Check sheet for the drawn part. Datum: minimum x, y, z corner. Units: mm. A direction names the side the tool comes from. Round coordinates to 2 decimals unless told otherwise and drop trailing zeros. Write each loop counter-clockwise with the first axis right and the second up, starting at its lowest first coordinate (ties: lowest second). Pieces come first, ordered by that corner, then holes.
Item 1: Cross-section at A-A on x = 12.75. Enter the section's corners in (y, z).
Item 2: Cross-section at B-B on z = 0.2. Enter the section's corners in (x, y).
Item 3: Tool access check on the marked faces 1 and 2. Record the directions out of +Z, -Z, +X, -X, +Y, -Y that give a thin tool (end or side, any length) a straight path to the whole face; none if there is none.
Item 4: Cross-section at C-C on y = 3.5. Enter the section's corners in (x, z).
Item 5: Release check for a two-part mould opening along Y. For the marked faces 3, 4 and 5 record: +Y half, -Y half, draft (parallel to the pull), parting line (faces both ways), or undercut.
Item 6: Cross-section at D-D on x = 9. Enter the section's corners in (y, z).
Item 7: Material ranges on line 1 (X direction, y = 11, z = 1.05); line 2 (Y direction, x = 12.5, z = 0.3); line 3 (Y direction, x = 8.25, z = 0.25), recorded low to high.
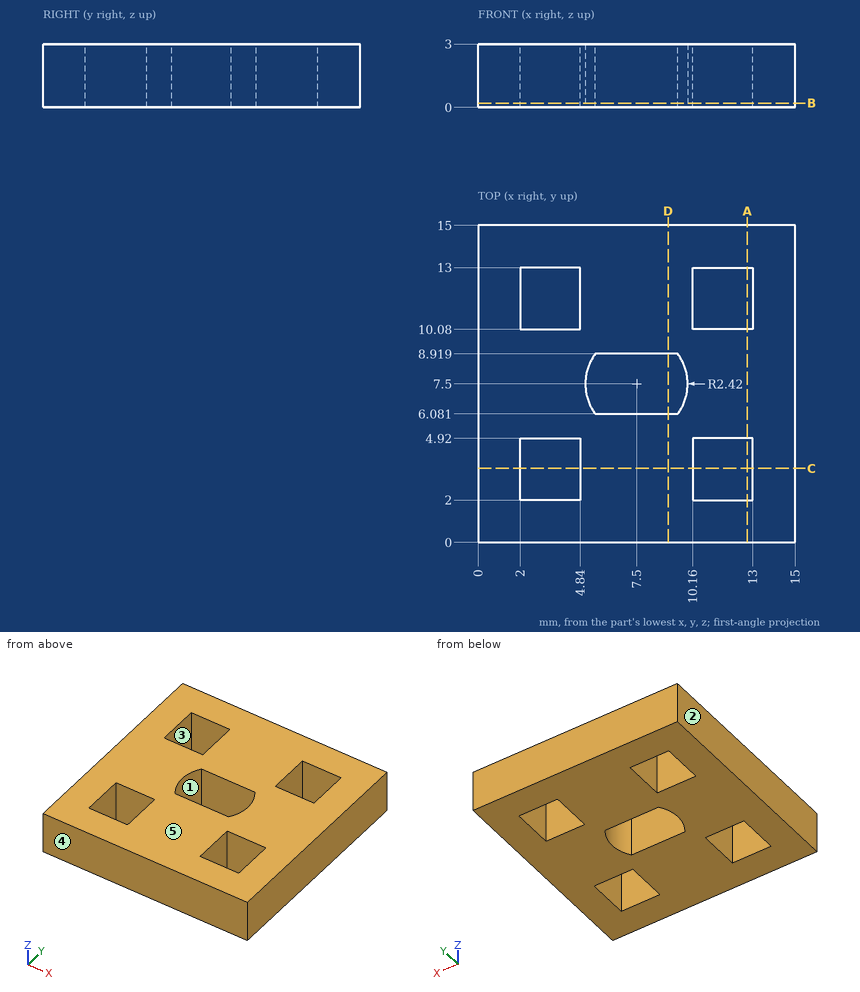
Response values:
1. outline: (0, 0) - (2, 0) - (2, 3) - (0, 3) - close; (4.92, 0) - (10.08, 0) - (10.08, 3) - (4.92, 3) - close; (13, 0) - (15, 0) - (15, 3) - (13, 3) - close
2. outline: (0, 0) - (15, 0) - (15, 15) - (0, 15) - close; hole (2, 2) - (4.84, 2) - (4.84, 4.92) - (2, 4.92) - close; hole (2, 10.08) - (4.84, 10.08) - (4.84, 13) - (2, 13) - close; hole (5.54, 6.08) - (9.46, 6.08) arc R2.42 ccw to (9.46, 8.92) - (5.54, 8.92) arc R2.42 ccw to start; hole (10.16, 2) - (13, 2) - (13, 4.92) - (10.16, 4.92) - close; hole (10.16, 10.08) - (13, 10.08) - (13, 13) - (10.16, 13) - close
3. face 1: +Z, -Z
3. face 2: +Z, -Z, -X, +Y, -Y
4. outline: (0, 0) - (2, 0) - (2, 3) - (0, 3) - close; (4.84, 0) - (10.16, 0) - (10.16, 3) - (4.84, 3) - close; (13, 0) - (15, 0) - (15, 3) - (13, 3) - close
5. face 3: undercut
5. face 4: -Y half
5. face 5: draft
6. outline: (0, 0) - (6.08, 0) - (6.08, 3) - (0, 3) - close; (8.92, 0) - (15, 0) - (15, 3) - (8.92, 3) - close
7. line 1: x = 0 to 2, 4.84 to 10.16, 13 to 15
7. line 2: y = 0 to 2, 4.92 to 10.08, 13 to 15
7. line 3: y = 0 to 6.08, 8.92 to 15
